Build history of the part. All positions in model axes, mm. Face numbers are marked on the shaded views. Give positions to 0.01 mm unless a question says otherwise; leave off trailing zeros. Loops run counter-clockwise (first coordinate to the right, second up) from the corner with the lowest first, then second, coordinate; pieces in that order, holes last. Notation, with made-up numbers: (82.25, 13) -> (110.25, 13) arc R30 ccw to (110.25, 44) -> close; hole circle Ø6 at (22.5, -27). An arc over 180 degrees is marked (long way). Answer as a JSON object with one key per item and string values. Group by question number.
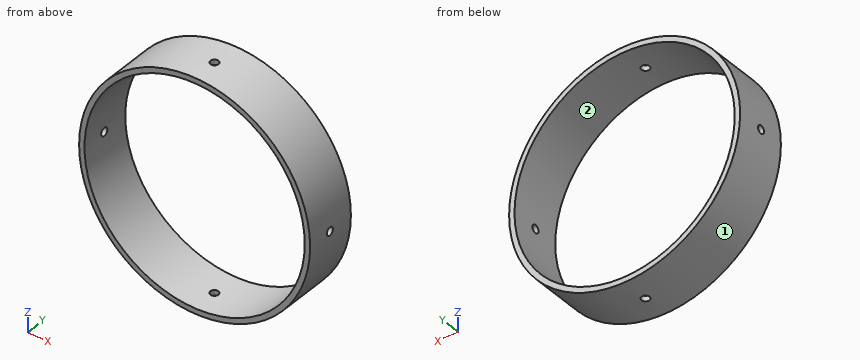
from build123d import *

# Parameters (mm, degrees)
SKETCH1_R           = 54.61
SKETCH1_R_2         = 52.07
BOSS_EXTRUDE1_DEPTH = 25.4
SKETCH3_R           = 1.905
CUT_EXTRUDE1_DEPTH  = 55.61
CIRPATTERN1_COUNT   = 4


with BuildPart() as part:
    # Sketch1 → Boss-Extrude1 (new body)
    with BuildSketch(Plane(origin=(0, 0, 0), x_dir=(1, 0, 0), z_dir=(0, 1, 0))):
        Circle(SKETCH1_R)
        Circle(SKETCH1_R_2, mode=Mode.SUBTRACT)
    extrude(amount=BOSS_EXTRUDE1_DEPTH)

    # Sketch3 → Cut-Extrude1 (cut, through all)
    with BuildSketch(Plane.XY):
        with Locations((0, 12.328955527)):
            Circle(SKETCH3_R)
    cut_extrude1 = extrude(amount=CUT_EXTRUDE1_DEPTH, mode=Mode.SUBTRACT)

    # CirPattern1: Cut-Extrude1 ×4 about axis
    cirpattern1_axis = Axis((0, 25.4, 0), (0, 1, 0))
    for i in range(1, CIRPATTERN1_COUNT):
        add(cut_extrude1.rotate(cirpattern1_axis, i * 360 / CIRPATTERN1_COUNT), mode=Mode.SUBTRACT)


solid = part.part
(1) Saw through at A-A on z = 0. List the corners of the cut face in (x, y).
(2) Saw through at D-D on x = -45. List the corners of the cut face in (y, z).
(3) Pull direction Z, two halves, no side cores. Call the marked faces 1 and 2: pulls with the +Z half, pulls with the -Z half, needs draft (parallel to the pull), parting line crosses it, or undercut.
(4) Saw through at B-B on x = 0. List the corners of the cut face in (y, z), plus the area to 3 significant figures.
(5) Probe line 1 along Y through (x, z) = (-53.3, 0); line 2 along X through (y, z) = (14.5, 0); line 3 along X through (y, z) = (21, 3). List the from-to ranges inside material, lowest first. Write a range as [from, to].
(6) Pin check, flat tips, straight feed: pin 1 (5 mm diameter, centred on x = -1.5, y = 22, fed in from -Z); pin 2 (5 mm diameter, centred on x = -25, y = 22, fed in from +Z); pin 3 (10 mm diameter, centred on x = -19, y = 17.5, fed in from -Z). Stop position of each tip, or through.
(7) Saw through at C-C on z = -14. List the corners of the cut face in (x, y).
Calculated:
{
 "1": {"outline": "(-54.61, 0) -> (-52.07, 0) -> (-52.07, 10.42) -> (-54.61, 10.42) -> close; (-54.61, 14.23) -> (-52.07, 14.23) -> (-52.07, 25.4) -> (-54.61, 25.4) -> close; (52.07, 0) -> (54.61, 0) -> (54.61, 10.42) -> (52.07, 10.42) -> close; (52.07, 14.23) -> (54.61, 14.23) -> (54.61, 25.4) -> (52.07, 25.4) -> close"},
 "2": {"outline": "(0, -30.94) -> (25.4, -30.94) -> (25.4, -26.2) -> (0, -26.2) -> close; (0, 26.2) -> (25.4, 26.2) -> (25.4, 30.94) -> (0, 30.94) -> close"},
 "3": {"face 1": "parting line crosses it", "face 2": "undercut"},
 "4": {"outline": "(0, -54.61) -> (10.42, -54.61) -> (10.42, -52.07) -> (0, -52.07) -> close; (0, 52.07) -> (10.42, 52.07) -> (10.42, 54.61) -> (0, 54.61) -> close; (14.23, -54.61) -> (25.4, -54.61) -> (25.4, -52.07) -> (14.23, -52.07) -> close; (14.23, 52.07) -> (25.4, 52.07) -> (25.4, 54.61) -> (14.23, 54.61) -> close", "area": "110 mm^2"},
 "5": {"line 1": "y = [0, 10.42], [14.23, 25.4]", "line 2": "x = [-54.61, -52.07], [52.07, 54.61]", "line 3": "x = [-54.53, -51.98], [51.98, 54.53]"},
 "6": {"pin 1": "stops at z = -54.61", "pin 2": "stops at z = 49.76", "pin 3": "stops at z = -52.78"},
 "7": {"outline": "(-52.78, 0) -> (-50.15, 0) -> (-50.15, 25.4) -> (-52.78, 25.4) -> close; (50.15, 0) -> (52.78, 0) -> (52.78, 25.4) -> (50.15, 25.4) -> close"}
}
